Part model, mm, in its own coordinate system. Round coordinates to 2 decimals unless told otherwise and drop trailing zeros. Write each loop counter-clockwise with the first axis right and the second up, starting at its lowest first coordinate (ties: lowest second). Pieces come first, ordered by that corner, then holes. Notation, with made-up numbers: M -34.75,79 L 24.25,79 A18 ccw 24.25,98 Z; hole C 74.5,30.25 d11. An arc over 180 degrees is marked long. Use a Markdown table: item, result. Add a question column.
1) Slice it at A-A on y = 17.75. Write the cut outline in (x, z), plus the area to 3 significant figures.
2) Slice it at B-B on x = 10. Write the cut outline in (y, z), plus the area to 3 significant figures.
3) Drop flat-ended pins along their axis: P1, Ø1, axis at x = 17.5, y = 14, coming from the -Z side; P2, Ø0.5, axis at y = 19, z = 9, coming from the +X side. Give the stop position or say it passes through.
4) Wall check: probe 1 along X at (y, z) = (13.25, -20.5); probe 2 along Y at (x, z) = (17.5, 23); probe 3 along X at (y, z) = (6.25, 21). Give the ranges that are in metal, low to high.
Autodesk Inventor part; units mm, degrees
ref_plane "Work Plane1" through (0, 0, 12.7) normal (0, 0, 1) x (1, 0, 0)
ref_plane "Work Plane2" through (1.5043, 20, 25.4) normal (0, 1, 0) x (1, 0, 0)
ref_plane "Work Plane3" through (10, 13.3333, 25.4) normal (-1, 0, 0) x (0, 0, 1)
sketch "Sketch1" plane through (0, 0, 0) normal (0, 0, 1) x (1, 0, 0)
  line L0 (11.2616, 7.5565) -> (11.8104, 7.0077)
  line L1 (11.8104, 7.0077) -> (12.9923, 8.1896)
  line L2 (12.9923, 8.1896) -> (12.4435, 8.7384)
  arc A0 (12.4435, 8.7384) -> (12.4435, 11.2616) centre (10, 10) ccw
  line L3 (12.4435, 11.2616) -> (12.9923, 11.8104)
  line L4 (12.9923, 11.8104) -> (11.8104, 12.9923)
  line L5 (11.8104, 12.9923) -> (11.2616, 12.4435)
  arc A1 (11.2616, 12.4435) -> (8.7384, 12.4435) centre (10, 10) ccw
  line L6 (8.7384, 12.4435) -> (8.1896, 12.9923)
  line L7 (8.1896, 12.9923) -> (7.0077, 11.8104)
  line L8 (7.0077, 11.8104) -> (7.5565, 11.2616)
  arc A2 (7.5565, 11.2616) -> (7.5565, 8.7384) centre (10, 10) ccw
  line L9 (7.5565, 8.7384) -> (7.0077, 8.1896)
  line L10 (7.0077, 8.1896) -> (8.1896, 7.0077)
  line L11 (8.1896, 7.0077) -> (8.7384, 7.5565)
  arc A3 (8.7384, 7.5565) -> (11.2616, 7.5565) centre (10, 10) ccw
  line L12 (13.4545, 0) -> (13.4545, 0.5)
  line L13 (13.4545, 0.5) -> (13, 0.5)
  line L14 (13, 0.5) -> (13, 1.5)
  line L15 (13, 1.5) -> (15.9091, 1.5)
  line L16 (15.9091, 1.5) -> (15.9091, 3)
  line L17 (15.9091, 3) -> (13.4545, 5.4545)
  line L18 (13.4545, 5.4545) -> (10.8302, 5.4545)
  arc A4 (10.8302, 5.4545) -> (9.1698, 5.4545) centre (10, 5.1837) ccw
  line L19 (9.1698, 5.4545) -> (6.6667, 5.4545)
  line L20 (6.6667, 5.4545) -> (4, 2.9545)
  line L21 (4, 2.9545) -> (4, 1.5909)
  line L22 (4, 1.5909) -> (7, 1.5909)
  line L23 (7, 1.5909) -> (7, 0.4545)
  line L24 (7, 0.4545) -> (6.6667, 0.4545)
  line L25 (6.6667, 0.4545) -> (6.6667, 0)
  line L26 (6.6667, 0) -> (1.5043, 0)
  arc A5 (0, 1.5043) -> (1.5043, 0) centre (1.5043, 1.5043) ccw
  line L27 (0, 1.5043) -> (0, 6.5455)
  line L28 (0, 6.5455) -> (0.5, 6.5455)
  line L29 (0.5, 6.5455) -> (0.5, 7)
  line L30 (0.5, 7) -> (1.5, 7)
  line L31 (1.5, 7) -> (1.5, 4.0909)
  line L32 (1.5, 4.0909) -> (3, 4.0909)
  line L33 (3, 4.0909) -> (5.4545, 6.5455)
  line L34 (5.4545, 6.5455) -> (5.4545, 9.1698)
  arc A6 (5.4545, 9.1698) -> (5.4545, 10.8302) centre (5.1837, 10) ccw
  line L35 (5.4545, 10.8302) -> (5.4545, 13.3333)
  line L36 (5.4545, 13.3333) -> (2.9545, 16)
  line L37 (2.9545, 16) -> (1.5909, 16)
  line L38 (1.5909, 16) -> (1.5909, 13)
  line L39 (1.5909, 13) -> (0.4545, 13)
  line L40 (0.4545, 13) -> (0.4545, 13.3333)
  line L41 (0.4545, 13.3333) -> (0, 13.3333)
  line L42 (0, 13.3333) -> (0, 18.4957)
  arc A7 (1.5043, 20) -> (0, 18.4957) centre (1.5043, 18.4957) ccw
  line L43 (1.5043, 20) -> (6.5455, 20)
  line L44 (6.5455, 20) -> (6.5455, 19.5)
  line L45 (6.5455, 19.5) -> (7, 19.5)
  line L46 (7, 19.5) -> (7, 18.5)
  line L47 (7, 18.5) -> (4.0909, 18.5)
  line L48 (4.0909, 18.5) -> (4.0909, 17)
  line L49 (4.0909, 17) -> (6.5455, 14.5455)
  line L50 (6.5455, 14.5455) -> (9.1698, 14.5455)
  arc A8 (9.1698, 14.5455) -> (10.8302, 14.5455) centre (10, 14.8163) ccw
  line L51 (10.8302, 14.5455) -> (13.3333, 14.5455)
  line L52 (13.3333, 14.5455) -> (16, 17.0455)
  line L53 (16, 17.0455) -> (16, 18.4091)
  line L54 (16, 18.4091) -> (13, 18.4091)
  line L55 (13, 18.4091) -> (13, 19.5455)
  line L56 (13, 19.5455) -> (13.3333, 19.5455)
  line L57 (13.3333, 19.5455) -> (13.3333, 20)
  line L58 (13.3333, 20) -> (18.4957, 20)
  arc A9 (20, 18.4957) -> (18.4957, 20) centre (18.4957, 18.4957) ccw
  line L59 (20, 18.4957) -> (20, 13.4545)
  line L60 (20, 13.4545) -> (19.5, 13.4545)
  line L61 (19.5, 13.4545) -> (19.5, 13)
  line L62 (19.5, 13) -> (18.5, 13)
  line L63 (18.5, 13) -> (18.5, 15.9091)
  line L64 (18.5, 15.9091) -> (17, 15.9091)
  line L65 (17, 15.9091) -> (14.5455, 13.4545)
  line L66 (14.5455, 13.4545) -> (14.5455, 10.8302)
  arc A10 (14.5455, 10.8302) -> (14.5455, 9.1698) centre (14.8163, 10) ccw
  line L67 (14.5455, 9.1698) -> (14.5455, 6.6667)
  line L68 (14.5455, 6.6667) -> (17.0455, 4)
  line L69 (17.0455, 4) -> (18.4091, 4)
  line L70 (18.4091, 4) -> (18.4091, 7)
  line L71 (18.4091, 7) -> (19.5455, 7)
  line L72 (19.5455, 7) -> (19.5455, 6.6667)
  line L73 (19.5455, 6.6667) -> (20, 6.6667)
  line L74 (20, 6.6667) -> (20, 1.5043)
  arc A11 (18.4957, 0) -> (20, 1.5043) centre (18.4957, 1.5043) ccw
  line L75 (18.4957, 0) -> (13.4545, 0)
  point P0 (0, 0)
  point P1 (0.4406, 0.4406)
  point P2 (10, 0)
  point P3 (10, 0)
  point P4 (10, 0)
  point P5 (19.5594, 0.4406)
  point P6 (0, 10)
  point P7 (0, 10)
  point P8 (0, 10)
  point P9 (10, 10)
  point P10 (20, 10)
  point P11 (20, 10)
  point P12 (20, 10)
  point P13 (0.4406, 19.5594)
  point P14 (10, 20)
  point P15 (10, 20)
  point P16 (10, 20)
  point P17 (19.5594, 19.5594)
extrude "Extrusion1" add sketch "Sketch1" along normal mid plane 50.8
ref_plane "Work Plane1" through (0, 0, 12.7) normal (0, 0, 1) x (1, 0, 0)
ref_plane "Work Plane2" through (1.5043, 20, 25.4) normal (0, 1, 0) x (1, 0, 0)
ref_plane "Work Plane3" through (10, 13.3333, 25.4) normal (-1, 0, 0) x (0, 0, 1)
properties part number "Verticle support"
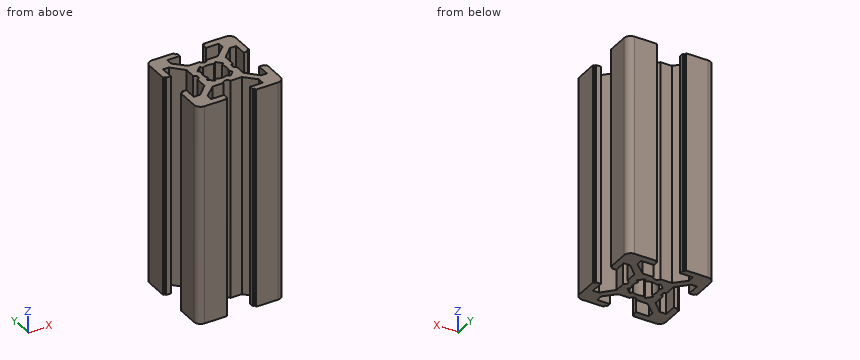
Entries:
| question | item | result |
|---|---|---|
| 1 | outline | M 0,-25.4 L 4.09,-25.4 L 4.09,25.4 L 0,25.4 Z; M 16,-25.4 L 20,-25.4 L 20,25.4 L 16,25.4 Z |
| 1 | area | 411 mm^2 |
| 2 | outline | M 6.06,-25.4 L 7.25,-25.4 L 7.25,25.4 L 6.06,25.4 Z; M 12.75,-25.4 L 13.94,-25.4 L 13.94,25.4 L 12.75,25.4 Z |
| 2 | area | 121 mm^2 |
| 3 | P1 | passes through |
| 3 | P2 | stops at x = 19.98 |
| 4 | probe 1 | x = 0.45 to 1.59, 5.45 to 14.55, 18.5 to 19.5 |
| 4 | probe 2 | y = 0 to 4, 15.91 to 20 |
| 4 | probe 3 | x = 0 to 1.5, 5.16 to 14.94, 18.41 to 20 |
